Source: CAD feature listing. Evaluate the final solid. Frame: model axes, mm. Face numbers are marked on the shaded views. A direction names the side the tool comes from. Round coordinates to 2 decimals unless told otherwise and drop trailing zeros. Order: outer loops, then holes, each group sorted by start corner. A loop starts at its lowest first (then second) coordinate and runs counter-clockwise, first axis right, second up. Notation, with made-up numbers: M 27,29 L 35,29 A19 cw 35,62 Z; hole C 24.25,60 d8. An arc over 180 degrees is marked long. Use one line per item in the form item = value. Start each with the question number.
Q1. Pull-direction query (Y, two-part tool) for the marked faces 3, 4 and 5; classes: pulls with the +Y half, pulls with the -Y half, needs draft (parallel to the pull), parting line crosses it, or undercut.
Q2. Section C-C (z = 30). Return the cut outline in (x, y), plus the area to 3 significant figures.
Q3. Section A-A (z = 2). Return the cut outline in (x, y) (3 decimals).
Q4. Material intervals for probe 1 along Y at (x, z) = (5.5, -21) (3 decimals); probe 2 along Z at (x, y) = (89, 83); probe 3 along Y at (x, z) = (84, 7), sorted ascending.
Q5. Section D-D (y = 54). Return the cut outline in (x, z).
Q6. Reachability of the marked faces 1 and 2 from +Z, -Z, +X, -X, +Y, -Y: full face, straight path, thin tool, end or side. Return the list, or none.
Q7. Section B-B (x = 109.5). Return the cut outline in (y, z) (1 decimal).
Q8. Contact query for flat-ended pins moving along their axis: pin 1 (3 mm diameter, centred on x = 42, y = 20.5, fed in from +Z); pin 2 (10 mm diameter, centred on x = 3.5, y = 64.5, fed in from -Z); pin 3 (5 mm diameter, centred on x = -12, y = 22.5, fed in from -Z). Output: stop coordinate, or through.
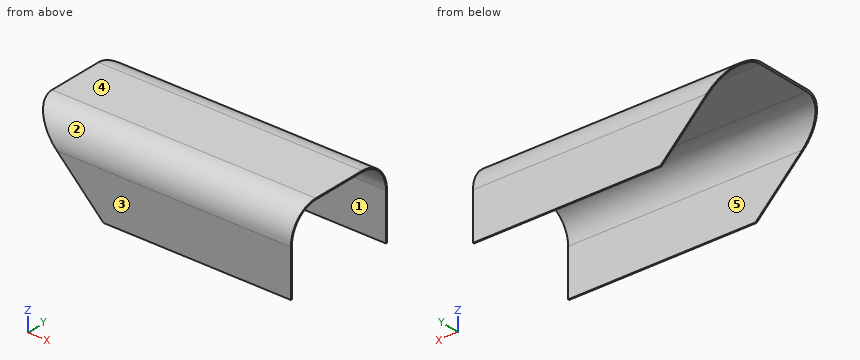
from build123d import *

# Parameters (mm, degrees)
BOSS_EXTRUDE1_DEPTH      = 196.85
BOSS_EXTRUDE1_DEPTH_BACK = 80.01
CUT_EXTRUDE1_DEPTH       = 196.85
CUT_EXTRUDE1_DEPTH_BACK  = 196.85


with BuildPart() as part:
    # Sketch1 → Boss-Extrude1 (new, two sides: drawn at the far end of the back side and taken through both)
    with BuildSketch(Plane(origin=(0, 0, -24.476668928), x_dir=(0, 0, -1), z_dir=(1, 0, 0)).offset(-BOSS_EXTRUDE1_DEPTH_BACK)):
        with BuildLine():
            Line((19.05, 118.745), (-30.1625, 118.745))
            ThreePointArc((-30.1625, 118.745), (-51.490608288, 109.910608288), (-60.325, 88.5825))
            Line((-60.325, 88.5825), (-60.325, 30.1625))
            ThreePointArc((-60.325, 30.1625), (-51.490608288, 8.834391712), (-30.1625, 0))
            Line((-30.1625, 0), (19.05, 0))
            Line((19.05, 0), (19.05, -1.27))
            Line((19.05, -1.27), (-30.1625, -1.27))
            ThreePointArc((-30.1625, -1.27), (-52.3886339, 7.9363661), (-61.595, 30.1625))
            Line((-61.595, 30.1625), (-61.595, 88.5825))
            ThreePointArc((-61.595, 88.5825), (-52.3886339, 110.8086339), (-30.1625, 120.015))
            Line((-30.1625, 120.015), (19.05, 120.015))
            Line((19.05, 120.015), (19.05, 118.745))
        make_face()
    extrude(amount=BOSS_EXTRUDE1_DEPTH + BOSS_EXTRUDE1_DEPTH_BACK)

    # Sketch2 → Cut-Extrude1 (cut, two sides: drawn at the far end of the back side and taken through both)
    with BuildSketch(Plane(origin=(0, 0, 0), x_dir=(1, 0, 0), z_dir=(0, 1, 0)).offset(-CUT_EXTRUDE1_DEPTH_BACK)):
        Polygon((0.210197293, 43.526668928), (-120.988442542, -78.530752949), (-120.988442542, 43.526668928), align=None)
    extrude(amount=CUT_EXTRUDE1_DEPTH + CUT_EXTRUDE1_DEPTH_BACK, mode=Mode.SUBTRACT)


solid = part.part
Results list:
q1.face_3 = pulls with the -Y half
q1.face_4 = needs draft
q1.face_5 = undercut
q2.outline = M -72.8,10.24 L 196.85,10.24 L 196.85,12.31 L -72.8,12.31 Z; M -72.8,106.43 L 196.85,106.43 L 196.85,108.5 L -72.8,108.5 Z
q2.area = 1,120 mm2
q3.outline = M -44.996,-1.27 L 196.85,-1.27 L 196.85,0 L -44.996,0 Z; M -44.996,118.745 L 196.85,118.745 L 196.85,120.015 L -44.996,120.015 Z
q4.probe_1 = -1.27 to 0, 118.745 to 120.015
q4.probe_2 = 35.85 to 37.12
q4.probe_3 = -1.24 to 0.03, 118.72 to 119.99
q5.outline = M -79.87,37.12 L -78.61,35.85 L 196.85,35.85 L 196.85,37.12 Z
q6.face_1 = -Z, +X, -X
q6.face_2 = +Z, +X, -X, -Y
q7.outline = M -1.3,-43.5 L 0,-43.5 L 0,5.7 A30.2 cw 30.2,35.8 L 88.6,35.8 A30.2 cw 118.7,5.7 L 118.7,-43.5 L 120,-43.5 L 120,5.7 A31.4 ccw 88.6,37.1 L 30.2,37.1 A31.4 ccw -1.3,5.7 Z
q8.pin_1 = 36.04
q8.pin_2 = 35.85
q8.pin_3 = 34.08
